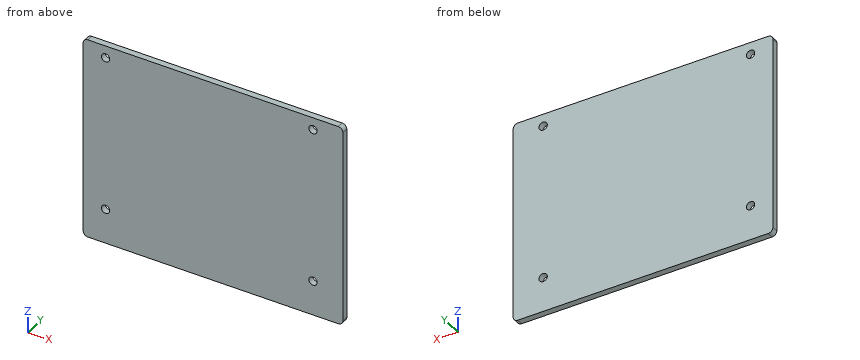
```python
from build123d import *

# Parameters (mm, degrees)
SKETCH_1_W          = 103
SKETCH_1_H          = 81
EXTRUDE_1_DEPTH     = 2.5
FILLET_1_R          = 2
SKETCH_2_R          = 1.65
CUT_EXTRUDE_1_DEPTH = 66.56485339
CUT_EXTRUDE_2_DEPTH = 66.56485339


with BuildPart() as part:
    # 草图1 → 凸台-拉伸1 (new body)
    with BuildSketch(Plane(origin=(0, 0, 0), x_dir=(1, 0, 0), z_dir=(0, 1, 0))):
        Rectangle(SKETCH_1_W, SKETCH_1_H)
    extrude(amount=EXTRUDE_1_DEPTH)

    # 圆角1
    fillet_1_edges = [part.edges().sort_by_distance(p)[0] for p in [
        (51.5, 1.25, 40.5),
        (-51.5, 1.25, 40.5),
        (-51.5, 1.25, -40.5),
        (51.5, 1.25, -40.5),
    ]]
    fillet(fillet_1_edges, radius=FILLET_1_R)

    # 草图2 → 切除-拉伸1 (cut, through all)
    with BuildSketch(Plane(origin=(0, 2.5, 0), x_dir=(1, 0, 0), z_dir=(0, 1, 0))):
        with Locations(Location((-42.5, 26.5, 0), (0, 0, 270))):
            Circle(SKETCH_2_R)
        with Locations(Location((39.5, 26.5, 0), (0, 0, 270))):
            Circle(SKETCH_2_R)
        with Locations(Location((39.5, -35.5, 0), (0, 0, 270))):
            Circle(SKETCH_2_R)
        with Locations(Location((-42.5, -35.5, 0), (0, 0, 270))):
            Circle(SKETCH_2_R)
    extrude(amount=-CUT_EXTRUDE_1_DEPTH, mode=Mode.SUBTRACT)

    # 草图3 → 切除-拉伸2 (cut, through all)
    with BuildSketch(Plane(origin=(0, 2.5, 0), x_dir=(1, 0, 0), z_dir=(0, 1, 0))):
        with BuildLine():
            Line((49.5, 40.5), (-49.5, 40.5))
            ThreePointArc((-49.5, 40.5), (-50.914213562, 39.914213562), (-51.5, 38.5))
            Line((-51.5, 38.5), (-51.5, -38.5))
            ThreePointArc((-51.5, -38.5), (-50.914213562, -39.914213562), (-49.5, -40.5))
            Line((-49.5, -40.5), (49.5, -40.5))
            ThreePointArc((49.5, -40.5), (50.914213562, -39.914213562), (51.5, -38.5))
            Line((51.5, -38.5), (51.5, 38.5))
            ThreePointArc((51.5, 38.5), (50.914213562, 39.914213562), (49.5, 40.5))
        make_face()
        with BuildLine():
            Line((49.5, 40.35), (-49.5, 40.35))
            ThreePointArc((-49.5, 40.35), (-50.808147545, 39.808147545), (-51.35, 38.5))
            Line((-51.35, 38.5), (-51.35, -38.5))
            ThreePointArc((-51.35, -38.5), (-50.808147545, -39.808147545), (-49.5, -40.35))
            Line((-49.5, -40.35), (49.5, -40.35))
            ThreePointArc((49.5, -40.35), (50.808147545, -39.808147545), (51.35, -38.5))
            Line((51.35, -38.5), (51.35, 38.5))
            ThreePointArc((51.35, 38.5), (50.808147545, 39.808147545), (49.5, 40.35))
        make_face(mode=Mode.SUBTRACT)
    extrude(amount=-CUT_EXTRUDE_2_DEPTH, mode=Mode.SUBTRACT)


solid = part.part
```
Read the model definition and answer for the solid it produces. Units are mm, in the model's axes. Coordinates: 2 decimals unless noted, no trailing zeros. Loops run counter-clockwise (first coordinate to the right, second up) from the corner with the lowest first, then second, coordinate; pieces in that order, holes last. Notation, with made-up numbers: (54, 47) -> (87, 47) arc R6 cw to (87, 53) -> close; hole circle Ø7 at (12, 62.5). An arc over 180 degrees is marked (long way). Return JSON: item names as keys, results as strings.
Item 1: Find the intervals of material crossed by probe 1 along X at (y, z) = (1.15, -26.5), in increasing order.
Answers:
{"probe 1": "x = -51.35 to -44.15, -40.85 to 37.85, 41.15 to 51.35"}
Item 2: A flat-ended cylindrical pin translates along its axis: P1, Ø3, axis at x = 13.5, z = -14, coming from the -Y side. Find the tip coordinate at first contact, or state that the pin passes through.
Answers:
{"P1": "stops at y = 0"}
Item 3: Find section B-B (x = -42.5). Determine the outline of the cut face in (y, z), plus the area to 3 significant figures.
Answers:
{"outline": "(0, -40.35) -> (2.5, -40.35) -> (2.5, -28.15) -> (0, -28.15) -> close; (0, -24.85) -> (2.5, -24.85) -> (2.5, 33.85) -> (0, 33.85) -> close; (0, 37.15) -> (2.5, 37.15) -> (2.5, 40.35) -> (0, 40.35) -> close", "area": "185 mm2"}
Item 4: Find section A-A (z = 35.5). Determine the outline of the cut face in (x, y).
Answers:
{"outline": "(-51.35, 0) -> (-44.15, 0) -> (-44.15, 2.5) -> (-51.35, 2.5) -> close; (-40.85, 0) -> (37.85, 0) -> (37.85, 2.5) -> (-40.85, 2.5) -> close; (41.15, 0) -> (51.35, 0) -> (51.35, 2.5) -> (41.15, 2.5) -> close"}
